```python
from build123d import *

# Parameters (mm, degrees)
F3_D     = 9.398
F3_DEPTH = 9.525
F3_TIP   = 2.8234440488
F5_D     = 3.19532
F5_DEPTH = 16.66875
F5_TIP   = 0.9599709766


with BuildPart() as f1:
    # F0 (on Front) → F1 (revolve)
    with BuildSketch(Plane.XZ):
        with BuildLine():
            Line((0, 22.8263996542), (0, -21.8741521218))
            Line((0, -21.8741521218), (2.54, -21.8741521218))
            add(Edge.make_bspline(
                [(2.54, -21.8741521218), (2.5441716884, -19.3644294307), (3.3400128786, -17.8042466392), (5.4864982158, -15.8082274963), (9.6622245064, -15.3927278895), (13.0963800475, -15.3518803418), (16.2190684, -15.3281874955)],
                knots=[0, 0, 0, 0, 0.2538500708, 0.4431641951, 0.6786842586, 1, 1, 1, 1], degree=3))
            Line((16.2190684, -15.3281874955), (23.8547402, -15.3281874955))
            ThreePointArc((23.8547402, -15.3281874955), (31.5188339477, -7.6640937477), (23.8547402, 0))
            Line((23.8547402, 0), (6.35, 0))
            Line((6.35, 0), (6.35, 6.35))
            Line((6.35, 6.35), (15.1027384, 6.35))
            ThreePointArc((15.1027384, 6.35), (20.3265735139, 11.5738351139), (15.1027384, 16.7976702278))
            Line((15.1027384, 16.7976702278), (6.35, 16.7976702278))
            Line((6.35, 16.7976702278), (6.35, 22.8263996542))
            Line((6.35, 22.8263996542), (0, 22.8263996542))
        make_face()
    revolve(axis=Axis((0, 0, 0.4761237662), (0, 0, -1)))

    # F3
    with Locations(Plane.XY.offset(22.8263996542)):
        with Locations((0, 0)):
            Hole(F3_D / 2, depth=F3_DEPTH)
            with Locations((0, 0, -(F3_DEPTH + F3_TIP / 2))):  # 118° drill point
                Cone(0, F3_D / 2, F3_TIP, mode=Mode.SUBTRACT)

    # F5
    with Locations(Plane(origin=(0, 0, -21.8741521218), x_dir=(1, 0, 0), z_dir=(0, 0, -1))):
        with Locations((0, 0)):
            Hole(F5_D / 2, depth=F5_DEPTH)
            with Locations((0, 0, -(F5_DEPTH + F5_TIP / 2))):  # 118° drill point
                Cone(0, F5_D / 2, F5_TIP, mode=Mode.SUBTRACT)


solid = f1.part
```
Part model, mm, in its own coordinate system. A direction names the side the tool comes from. Round coordinates to 2 decimals unless told otherwise and drop trailing zeros. Order: outer loops, then holes, each group sorted by start corner. A loop starts at its lowest first (then second) coordinate and runs counter-clockwise, first axis right, second up. Notation, with made-up numbers: M -21.5,61 L -9.5,61 A13 cw -9.5,74 Z; hole C 83.5,-0.5 d9. An arc over 180 degrees is marked long. Answer in a Markdown table with one row per item. Add a question column.
Q1. Cut at B-B on z = 9. Give the cut face in (x, y).
Q2. Pin check, flat tips, straight feed: pin 1 (3 mm diameter, centred on y = -4, z = 8, fed in from -X); pin 2 (3 mm diameter, centred on y = 21.5, z = 16.5, fed in from +X); pin 3 (2 mm diameter, centred on x = 4.5, y = 7.5, fed in from +Z); pin 4 (10 mm diameter, centred on x = 3, y = 23, fed in from -Z). Stop position of each tip, or through.
Q3. Cut at A-A on z = -13. Give the cut face in (x, y), and give its area (3 significant figures).
Q4. Mould opens along Z. For faces 4 (the face through (0, -5, 22.826)), 5 (the face through (-0.06, 0.27, -4.41)), 6 (the face through (-1.38, 6.2, 3.22)) say: +Z half, -Z half, draft (parallel to the pull), parting line (faces both ways), or undercut.
Q5. Wall check: L1, parallel to X at y = 0, z = 18; L2, parallel to Z at x = 9.5, y = -18; L3, parallel to Z at x = -7.5, y = -1. Give the ranges that are in metal, low to high. Write a range as from..to.
Q6. 3-axis set-ups, long thin cutter, end or side, ignore diameter. For faces 1 (the face through (0, 7, 6.35)), 2 (the face through (-1.38, 6.2, 19.85)), 3 (the face through (0.208, -1.584, -13.423)): which of +Z, -Z, +X, -X, +Y, -Y reach the whole face in a straight line?
Established:
| question | item | result |
|---|---|---|
| 1 | outline | C 0,0 d39.3 |
| 2 | pin 1 | stops at x = -19.55 |
| 2 | pin 2 | passes through |
| 2 | pin 3 | stops at z = 16.8 |
| 2 | pin 4 | stops at z = -15.33 |
| 3 | outline | C 0,0 d58.71; hole C 0,0 d3.2 |
| 3 | area | 2,700 mm2 |
| 4 | face 4 | +Z half |
| 4 | face 5 | -Z half |
| 4 | face 6 | undercut |
| 5 | L1 | x = -6.35..-4.7, 4.7..6.35 |
| 5 | L2 | z = -15.33..0 |
| 5 | L3 | z = -15.64..0, 6.35..16.8 |
| 6 | face 1 | none |
| 6 | face 2 | +Z |
| 6 | face 3 | -Z |
